```python
from build123d import *

# Parameters (mm, degrees)
MODEL_R             = 3
BOSS_EXTRUDE1_DEPTH = 4


with BuildPart() as part:
    # Model → Boss-Extrude1 (new body)
    with BuildSketch(Plane.XY):
        with BuildLine():
            Line((220, -99.8), (220, -74.9))
            Line((220, -74.9), (160.3, -55))
            Line((160.3, -55), (49, -55))
            ThreePointArc((49, -55), (47.585786438, -55.585786438), (47, -57))
            Line((47, -57), (47, -69))
            ThreePointArc((47, -69), (46.414213562, -70.414213562), (45, -71))
            Line((45, -71), (27, -71))
            ThreePointArc((27, -71), (25.585786438, -70.414213562), (25, -69))
            Line((25, -69), (25, -57))
            ThreePointArc((25, -57), (24.414213562, -55.585786438), (23, -55))
            Line((23, -55), (-23, -55))
            ThreePointArc((-23, -55), (-24.414213562, -55.585786438), (-25, -57))
            Line((-25, -57), (-25, -69))
            ThreePointArc((-25, -69), (-25.585786438, -70.414213562), (-27, -71))
            Line((-27, -71), (-45, -71))
            ThreePointArc((-45, -71), (-46.414213562, -70.414213562), (-47, -69))
            Line((-47, -69), (-47, -57))
            ThreePointArc((-47, -57), (-47.585786438, -55.585786438), (-49, -55))
            Line((-49, -55), (-168, -55))
            ThreePointArc((-168, -55), (-169.414213562, -54.414213562), (-170, -53))
            Line((-170, -53), (-170, 53))
            ThreePointArc((-170, 53), (-169.414213562, 54.414213562), (-168, 55))
            Line((-168, 55), (-49, 55))
            ThreePointArc((-49, 55), (-47.585786438, 55.585786438), (-47, 57))
            Line((-47, 57), (-47, 69))
            ThreePointArc((-47, 69), (-46.414213562, 70.414213562), (-45, 71))
            Line((-45, 71), (-27, 71))
            ThreePointArc((-27, 71), (-25.585786438, 70.414213562), (-25, 69))
            Line((-25, 69), (-25, 55))
            Line((-25, 55), (23, 55))
            ThreePointArc((23, 55), (24.414213562, 55.585786438), (25, 57))
            Line((25, 57), (25, 69))
            ThreePointArc((25, 69), (25.585786438, 70.414213562), (27, 71))
            Line((27, 71), (45, 71))
            ThreePointArc((45, 71), (46.414213562, 70.414213562), (47, 69))
            Line((47, 69), (47, 57))
            ThreePointArc((47, 57), (47.585786438, 55.585786438), (49, 55))
            Line((49, 55), (160.3, 55))
            Line((160.3, 55), (220, 74.9))
            Line((220, 74.9), (220, 99.8))
            Line((220, 99.8), (195, 99.8))
            Line((195, 99.8), (195, 125))
            Line((195, 125), (-195, 125))
            Line((-195, 125), (-195, 99.8))
            Line((-195, 99.8), (-220, 99.8))
            Line((-220, 99.8), (-220, -99.8))
            Line((-220, -99.8), (-195, -99.8))
            Line((-195, -99.8), (-195, -125))
            Line((-195, -125), (195, -125))
            Line((195, -125), (195, -99.8))
            Line((195, -99.8), (220, -99.8))
        make_face()
        with Locations((36, 80)):
            Circle(MODEL_R, mode=Mode.SUBTRACT)
        with Locations((-36, -80)):
            Circle(MODEL_R, mode=Mode.SUBTRACT)
        with Locations((-36, 80)):
            Circle(MODEL_R, mode=Mode.SUBTRACT)
        with Locations((36, -80)):
            Circle(MODEL_R, mode=Mode.SUBTRACT)
        with Locations((55, 112.5)):
            Circle(MODEL_R, mode=Mode.SUBTRACT)
        with Locations((-110, 112.5)):
            Circle(MODEL_R, mode=Mode.SUBTRACT)
        with Locations((-55, 112.5)):
            Circle(MODEL_R, mode=Mode.SUBTRACT)
        with Locations((0, 112.5)):
            Circle(MODEL_R, mode=Mode.SUBTRACT)
        with Locations((-165, 112.5)):
            Circle(MODEL_R, mode=Mode.SUBTRACT)
        with Locations((110, 112.5)):
            Circle(MODEL_R, mode=Mode.SUBTRACT)
        with Locations((165, 112.5)):
            Circle(MODEL_R, mode=Mode.SUBTRACT)
        with Locations((110, -112.5)):
            Circle(MODEL_R, mode=Mode.SUBTRACT)
        with Locations((-165, -112.5)):
            Circle(MODEL_R, mode=Mode.SUBTRACT)
        with Locations((0, -112.5)):
            Circle(MODEL_R, mode=Mode.SUBTRACT)
        with Locations((-55, -112.5)):
            Circle(MODEL_R, mode=Mode.SUBTRACT)
        with Locations((-110, -112.5)):
            Circle(MODEL_R, mode=Mode.SUBTRACT)
        with Locations((55, -112.5)):
            Circle(MODEL_R, mode=Mode.SUBTRACT)
        with Locations((165, -112.5)):
            Circle(MODEL_R, mode=Mode.SUBTRACT)
        with BuildLine():
            Line((170, -83), (100, -83))
            ThreePointArc((100, -83), (97, -80), (100, -77))
            Line((100, -77), (170, -77))
            ThreePointArc((170, -77), (173, -80), (170, -83))
        make_face(mode=Mode.SUBTRACT)
        with BuildLine():
            Line((-170, -77), (-100, -77))
            ThreePointArc((-100, -77), (-97, -80), (-100, -83))
            Line((-100, -83), (-170, -83))
            ThreePointArc((-170, -83), (-173, -80), (-170, -77))
        make_face(mode=Mode.SUBTRACT)
        with BuildLine():
            Line((170, 77), (100, 77))
            ThreePointArc((100, 77), (97, 80), (100, 83))
            Line((100, 83), (170, 83))
            ThreePointArc((170, 83), (173, 80), (170, 77))
        make_face(mode=Mode.SUBTRACT)
        with BuildLine():
            Line((-170, 83), (-100, 83))
            ThreePointArc((-100, 83), (-97, 80), (-100, 77))
            Line((-100, 77), (-170, 77))
            ThreePointArc((-170, 77), (-173, 80), (-170, 83))
        make_face(mode=Mode.SUBTRACT)
    extrude(amount=BOSS_EXTRUDE1_DEPTH)


solid = part.part
```
The model under review builds one solid part; all positions refer to its coordinate system, in mm. A direction names the side the tool comes from. Round coordinates to 2 decimals unless told otherwise and drop trailing zeros. Loops run counter-clockwise (first coordinate to the right, second up) from the corner with the lowest first, then second, coordinate; pieces in that order, holes last. Notation, with made-up numbers: (-4, 60) -> (11, 60) arc R19 cw to (11, 65) -> close; hole circle Ø2 at (-6, 85). An arc over 180 degrees is marked (long way). Answer in a Markdown table with one row per item.
1) Draft analysis for pull direction Y (two halves, no side actions). For faces 1 (the flat face through (-3, 57, 4)), 2 (the flat face through (190.6, -65.1, 2)), state which applies: pulls with the +Y half, pulls with the -Y half, needs draft (parallel to the pull), parting line crosses it, or undercut.
Taken from the geometry:
| item | result |
|---|---|
| face 1 | needs draft |
| face 2 | undercut |
2) Consider section C-C, the plane z = 2.1. Count the separate pieces of the cut face and the enclosed holes in it, plus the area to 3 significant figures.
Taken from the geometry:
| item | result |
|---|---|
| separate pieces | 1 |
| enclosed holes | 22 |
| area | 59,700 mm² |
3) Consider section D-D, the plane y = 27. Write out the cut boundary in (x, z).
Taken from the geometry:
| item | result |
|---|---|
| outline | (-220, 0) -> (-170, 0) -> (-170, 4) -> (-220, 4) -> close |
4) Consider section B-B, the plane x = -71. Write out the cut boundary in (y, z), plus the area to 3 significant figures.
Taken from the geometry:
| item | result |
|---|---|
| outline | (-125, 0) -> (-55, 0) -> (-55, 4) -> (-125, 4) -> close; (55, 0) -> (125, 0) -> (125, 4) -> (55, 4) -> close |
| area | 560 mm² |
5) Tool access review of faces 3 (the flat face through (-3, 57, 0)), 4 (the flat face through (189.7, 64.8, 2)): name each direction out of +Z, -Z, +X, -X, +Y, -Y from which nothing blocks a thin tool from reaching the whole face with its end or side.
Taken from the geometry:
| item | result |
|---|---|
| face 3 | -Z, +X, -X, +Y, -Y |
| face 4 | +Z, -Z, +X |
6) Consider section A-A, the plane x = -140.5. Write out the cut boundary in (y, z), plus the area to 3 significant figures.
Taken from the geometry:
| item | result |
|---|---|
| outline | (-125, 0) -> (-83, 0) -> (-83, 4) -> (-125, 4) -> close; (-77, 0) -> (-55, 0) -> (-55, 4) -> (-77, 4) -> close; (55, 0) -> (77, 0) -> (77, 4) -> (55, 4) -> close; (83, 0) -> (125, 0) -> (125, 4) -> (83, 4) -> close |
| area | 512 mm² |
7) Wall thickness on line 1 along Y through (x, z) = (-55, 2.1); line 2 along Y through (x, z) = (-142, 2); line 3 along Y through (x, z) = (-40, 3.3): over which ranges is each line inside the solid? List them lowest first.
Taken from the geometry:
| item | result |
|---|---|
| line 1 | y = -125 to -115.5, -109.5 to -55, 55 to 109.5, 115.5 to 125 |
| line 2 | y = -125 to -83, -77 to -55, 55 to 77, 83 to 125 |
| line 3 | y = -125 to -71, 71 to 125 |
